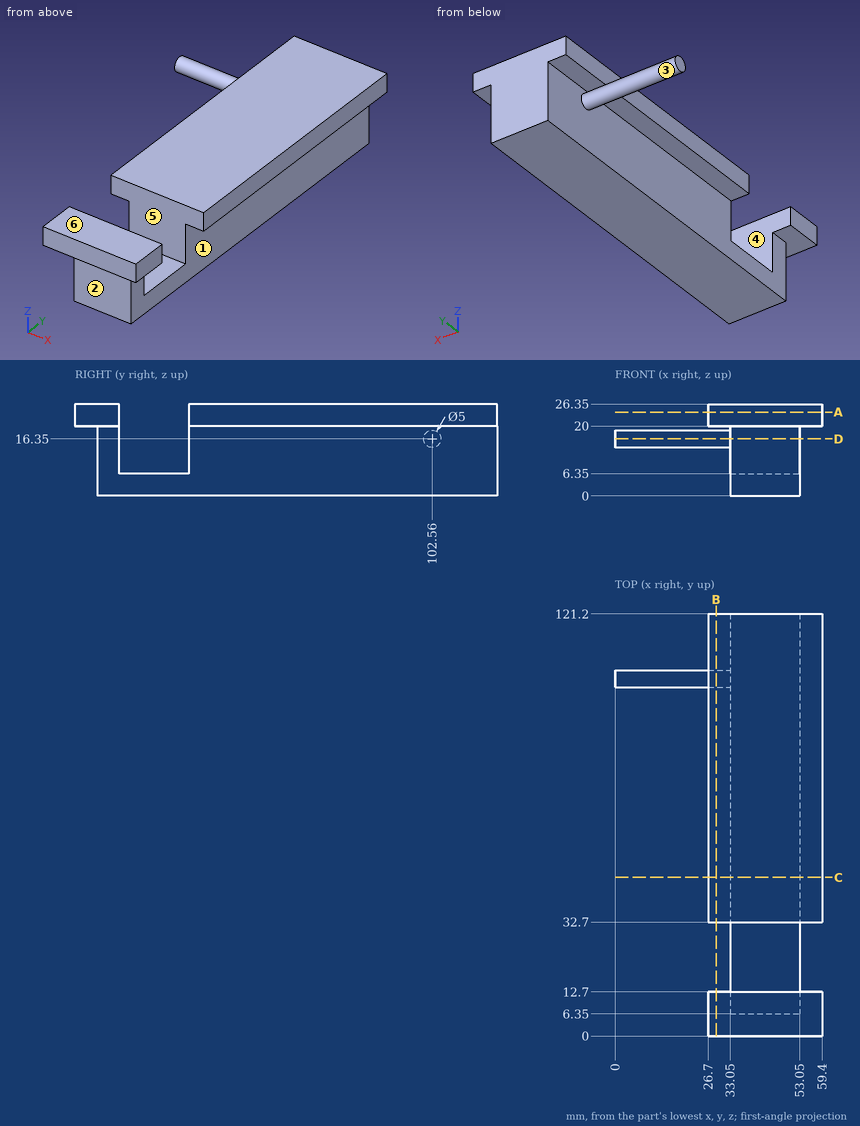
Can you work these out from the drawing? Everything is in mm from the part's minimum corner. A direction names the side the tool comes from. Give positions to 0.01 mm unless a question says otherwise; leave off trailing zeros. Order: outer loops, then holes, each group sorted by start corner. A loop starts at its lowest first (then second) coordinate and runs counter-clockwise, first axis right, second up. Notation, with made-up numbers: M 72,13.25 L 88,13.25 A11 ccw 88,20.25 Z; hole C -23,-2 d6. An arc over 180 degrees is marked long. One line per item, written item: value.
Item 1: For pin 1 (1 mm diameter, centred on x = 30, y = 80.5, fed in from -Z); pin 2 (4 mm diameter, centred on y = 53, z = 12.5, fed in from -X); pin 3 (1.5 mm diameter, centred on y = 50, z = 15, fed in from +X); pin 4 (3 mm diameter, centred on x = 15.5, z = 21.5, fed in from -Y), each with a flat end and sliding along its axis, tell me the tip position at first contact or that it passes through.
Verdict:
pin 1: z = 20
pin 2: x = 33.05
pin 3: x = 53.05
pin 4: through
Item 2: If we section it at A-A on z = 24: Write out the boundary of the cut face in (x, y), and give its area (3 significant figures).
Verdict:
outline: M 26.7,0 L 59.4,0 L 59.4,12.7 L 26.7,12.7 Z; M 26.7,32.7 L 59.4,32.7 L 59.4,121.2 L 26.7,121.2 Z
area: 3,310 mm2
Item 3: Please list where these lines run through material, in increasing order: line 1 (Y direction, x = 48, z = 17.75); line 2 (X direction, y = 97, z = 1.75); line 3 (Y direction, x = 31, z = 16).
Verdict:
line 1: 6.35 to 12.7, 32.7 to 121.2
line 2: 33.05 to 53.05
line 3: 100.08 to 105.04
Item 4: For the marked faces 5 and 6, which set-ups out of +Z, -Z, +X, -X, +Y, -Y let a thin tool reach every point of the face, with its end or its side?
Verdict:
face 5: +Z, +X, -X
face 6: +Z, +X, -X, +Y, -Y
Item 5: If we section it at D-D on z = 16.35: Write out the boundary of the cut face in (x, y).
Verdict:
outline: M 0,100.06 L 33.05,100.06 L 33.05,32.7 L 53.05,32.7 L 53.05,121.2 L 33.05,121.2 L 33.05,105.06 L 0,105.06 Z; M 33.05,6.35 L 53.05,6.35 L 53.05,12.7 L 33.05,12.7 Z
Item 6: If we section it at B-B on x = 29: Write out the boundary of the cut face in (y, z), and give its area (3 significant figures).
Verdict:
outline: M 0,20 L 12.7,20 L 12.7,26.35 L 0,26.35 Z; M 32.7,20 L 121.2,20 L 121.2,26.35 L 32.7,26.35 Z; C 102.56,16.35 d5
area: 662 mm2
Item 7: If we mould it in two halves opening along Y, with no side actions, what happens to the marked faces 1, 2, 3 and 4? For each: pulls with the +Y half, pulls with the -Y half, needs draft (parallel to the pull), parting line crosses it, or undercut.
Verdict:
face 1: needs draft
face 2: pulls with the -Y half
face 3: parting line crosses it
face 4: undercut
Item 8: If we section it at C-C on y = 45.5: Write out the boundary of the cut face in (x, z).
Verdict:
outline: M 26.7,20 L 33.05,20 L 33.05,0 L 53.05,0 L 53.05,20 L 59.4,20 L 59.4,26.35 L 26.7,26.35 Z
